Geometry check sheet. Reference: the model listing, model coordinates, mm. Face numbers are marked on the shaded views. A direction names the side the tool comes from. Give positions to 0.01 mm unless a question says otherwise; leave off trailing zeros. Order: outer loops, then holes, each group sorted by start corner. A loop starts at its lowest first (then second) coordinate and runs counter-clockwise, first axis right, second up. Notation, with made-up numbers: M 36,10.25 L 72,10.25 A15 ccw 72,35.25 Z; hole C 63,59 d7. An arc over 180 degrees is marked long. Put each result on its own line as item: value. Start each with the question number.
Q1. Material ranges on L1, parallel to Y at x = 40, z = -113.75; L2, parallel to Z at x = 8, y = -5.25; L3, parallel to Y at x = 14, z = -23, recorded low to high.
Q2. Section check C-C on y = -20. Record the cut outline in (x, z), then the cut area to 3 significant figures.
Q3. Access from +Z, -Z, +X, -X, +Y, -Y to the whole of each face (thin tool, end or side, straight path). Record for the marked faces 1 and 2.
Q4. Go/stop test with flat-tipped pins: pin 1 (7 mm diameter, centred on x = 10, y = -20, fed in from +Z); pin 2 (6 mm diameter, centred on x = 26, y = -14.5, fed in from +Z); pin 3 (25 mm diameter, centred on x = 31.5, z = -66, fed in from -Y). Record where each tip stops, or that it passes through.
Q5. Section check D-D on z = -113. Record the cut outline in (x, y), then the cut area to 3 significant figures.
Q6. Section check B-B on x = 8. Record the cut outline in (y, z), then the cut area to 3 significant figures.
Q7. Section check A-A on z = -42. Record the cut outline in (x, y), then the cut area to 3 significant figures.
```python
from build123d import *

# Parameters (mm, degrees)
F0_W     = 50
F0_H     = 120
F1_DEPTH = 10
F2_W     = 50
F2_H     = 10
F3_DEPTH = 20
F4_R     = 4.5
F5_DEPTH = 10.001
F7_D     = 4.2


with BuildPart() as f1:
    # F0 (on Front) → F1 (new body)
    with BuildSketch(Plane.XZ):
        with Locations((25, -60)):
            Rectangle(F0_W, F0_H)
    extrude(amount=F1_DEPTH)

    # F2 (on face) → F3 (join)
    with BuildSketch(Plane.XZ.offset(10)):
        with Locations((25, -115)):
            Rectangle(F2_W, F2_H)
    extrude(amount=F3_DEPTH)

    # F4 (on face) → F5 (cut, through all)
    with BuildSketch(Plane.XY.offset(-110)):
        with Locations((10, -20)):
            Circle(F4_R)
        with Locations((40, -20)):
            Circle(F4_R)
    extrude(amount=-F5_DEPTH, mode=Mode.SUBTRACT)

    # F7 (through all)
    with Locations(Plane.XZ.offset(10)):
        with Locations((8, -8), (42, -42)):
            Hole(F7_D / 2)


solid = f1.part
```
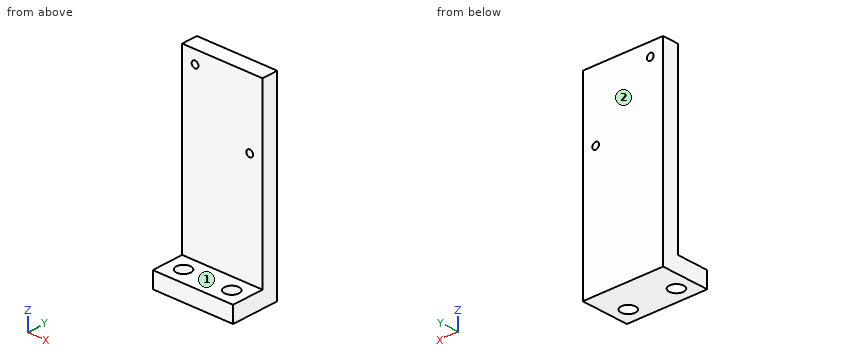
Results found:
1. L1: y = -30 to -24.5, -15.5 to 0
1. L2: z = -120 to -10.1, -5.9 to 0
1. L3: y = -10 to 0
2. outline: M 0,-120 L 5.5,-120 L 5.5,-110 L 0,-110 Z; M 14.5,-120 L 35.5,-120 L 35.5,-110 L 14.5,-110 Z; M 44.5,-120 L 50,-120 L 50,-110 L 44.5,-110 Z
2. area: 320 mm^2
3. face 1: +Z, +X, -X, -Y
3. face 2: +Z, -Z, +X, -X, +Y
4. pin 1: passes through
4. pin 2: stops at z = -110
4. pin 3: stops at y = -10
5. outline: M 0,-30 L 50,-30 L 50,0 L 0,0 Z; hole C 10,-20 d9; hole C 40,-20 d9
5. area: 1,370 mm^2
6. outline: M -30,-120 L -24.03,-120 L -24.03,-110 L -30,-110 Z; M -15.97,-120 L 0,-120 L 0,-10.1 L -10,-10.1 L -10,-110 L -15.97,-110 Z; M -10,-5.9 L 0,-5.9 L 0,0 L -10,0 Z
6. area: 1,280 mm^2
7. outline: M 0,-10 L 39.9,-10 L 39.9,0 L 0,0 Z; M 44.1,-10 L 50,-10 L 50,0 L 44.1,0 Z
7. area: 458 mm^2
